CAD build for the part. Positions are in the model's coordinates, mm. Give positions to 0.01 mm unless a question says otherwise; leave off trailing zeros. Write each loop counter-clockwise with the first axis right and the second up, starting at its lowest first coordinate (ties: lowest second). Pieces come first, ordered by that corner, then holes. Notation, with made-up numbers: (6.5, 82) - (32.5, 82) arc R31 cw to (32.5, 112) - close; hole circle Ø1 at (25, -36). An arc over 180 degrees is marked (long way). Answer as a JSON object with one key per item and string values.
from build123d import *

# Parameters (mm, degrees)
EXTRUDE_1_DEPTH     = 2
SKETCH_2_R          = 2
CUT_EXTRUDE_1_DEPTH = 2


with BuildPart() as part:
    # 草图1 → 凸台-拉伸1 (new body)
    with BuildSketch(Plane(origin=(0, 0, 0), x_dir=(1, 0, 0), z_dir=(0, 1, 0))):
        with BuildLine():
            Line((-4.507909161, 0), (-1.477242174, -16.275084839))
            ThreePointArc((-1.477242174, -16.275084839), (0.138127237, -17.496274365), (1.502636386, -16))
            Line((1.502636386, -16), (4.507909161, 0))
            ThreePointArc((4.507909161, 0), (0, 4.507909161), (-4.507909161, 0))
        make_face()
    extrude(amount=EXTRUDE_1_DEPTH)

    # 草图2 → 切除-拉伸1 (cut)
    with BuildSketch(Plane(origin=(0, 2, 0), x_dir=(1, 0, 0), z_dir=(0, 1, 0))):
        Circle(SKETCH_2_R)
    extrude(amount=-CUT_EXTRUDE_1_DEPTH, mode=Mode.SUBTRACT)


solid = part.part
(1) Flat gauge pin, fed straight in: P1, Ø2.5, axis at x = 0, z = 0, coming from the -Y side. Where does the tip first touch, or does it go through?
Answer key:
{"P1": "passes through"}
(2) Saw through at D-D, the plane z = 9.75. Give the cut face in (x, y).
Answer key:
{"outline": "(-2.69, 0) - (2.68, 0) - (2.68, 2) - (-2.69, 2) - close"}
(3) Saw through at C-C, the plane z = 1.5. Give the cut face in (x, y).
Answer key:
{"outline": "(-4.23, 0) - (-1.32, 0) - (-1.32, 2) - (-4.23, 2) - close; (1.32, 0) - (4.23, 0) - (4.23, 2) - (1.32, 2) - close"}
(4) Probe L1, parallel to Z at x = 0, y = 1; L2, parallel to Z at x = -1.25, y = 1.45; L3, parallel to X at y = 0.7, z = -0.25. List the from-to ranges inside material, lowest first. Write a range as [from, to].
Answer key:
{"L1": "z = [-4.51, -2], [2, 17.5]", "L2": "z = [-4.33, -1.56], [1.56, 16.83]", "L3": "x = [-4.5, -1.98], [1.98, 4.5]"}
(5) Saw through at A-A, the plane x = 0. Give the cut face in (y, z).
Answer key:
{"outline": "(0, -4.51) - (2, -4.51) - (2, -2) - (0, -2) - close; (0, 2) - (2, 2) - (2, 17.5) - (0, 17.5) - close"}
(6) Saw through at B-B, the plane y = 1.6. Give the cut face in (x, z).
Answer key:
{"outline": "(-4.51, 0) arc R4.51 ccw to (4.51, 0) - (1.5, 16) arc R1.5 ccw to (-1.48, 16.28) - close; hole circle Ø4 at (0, 0)"}
(7) Pull direction X, two halves, no side cores. Call faces 1 (the face through (0, 2, 6)), 2 (the face through (0, 1, 2)), 3 (the face through (0.099, 0.986, -4.507)): pulls with the +X half, pulls with the -X half, needs draft (parallel to the pull), parting line crosses it, or undercut.
Answer key:
{"face 1": "needs draft", "face 2": "undercut", "face 3": "parting line crosses it"}
